The listing builds one solid part. Answer for the finished solid, in the listing's coordinates (mm). A direction names the side the tool comes from. Give positions to 0.01 mm unless a question says otherwise; leave off trailing zeros. Order: outer loops, then holes, each group sorted by start corner. A loop starts at its lowest first (then second) coordinate and runs counter-clockwise, first axis right, second up. Notation, with made-up numbers: (-28.5, -4) -> (16.5, -4) arc R22 cw to (16.5, 2) -> close; hole circle Ø8 at (69, 32.5). An arc over 180 degrees is marked (long way). Answer as a JSON object with one key per item and string values. Group by question number.
```python
from build123d import *

# Parameters (mm, degrees)
SKETCH1_W               = 203.2
SKETCH1_H               = 152.4
BOSS_EXTRUDE2_DEPTH     = 5.334
SKETCH2_R               = 17.5
CUT_EXTRUDE1_DEPTH      = 184.239656068
SKETCH3_W               = 24.13
SKETCH3_H               = 5.08
BOSS_EXTRUDE3_DEPTH     = 5.334
SKETCH4_W               = 5.842
SKETCH4_H               = 12.954
CUT_EXTRUDE2_DEPTH      = 184.239656068
MIRROR3_COPY_1_SKETCH_W = 24.13
MIRROR3_COPY_1_SKETCH_H = 5.08
MIRROR3_COPY_1_DEPTH    = 5.334


with BuildPart() as part:
    # Sketch1 → Boss-Extrude2 (new body)
    with BuildSketch(Plane(origin=(0, 0, 0), x_dir=(0, 0, -1), z_dir=(1, 0, 0))):
        with Locations((0, 76.2)):
            Rectangle(SKETCH1_W, SKETCH1_H)
    extrude(amount=BOSS_EXTRUDE2_DEPTH)

    # Sketch2 → Cut-Extrude1 (cut, through all)
    with BuildSketch(Plane.ZY):
        with Locations((0, 76.2)):
            Circle(SKETCH2_R)
    extrude(amount=-CUT_EXTRUDE1_DEPTH, mode=Mode.SUBTRACT)

    # Sketch3 → Boss-Extrude3 (add, through all)
    with BuildSketch(Plane.ZY):
        with Locations((69.85, -2.54)):
            Rectangle(SKETCH3_W, SKETCH3_H)
    boss_extrude3 = extrude(amount=-BOSS_EXTRUDE3_DEPTH)

    # Mirror1: Boss-Extrude3 across plane
    add(boss_extrude3.mirror(Plane.XY))

    # Sketch4 → Cut-Extrude2 (cut, through all)
    with BuildSketch(Plane.ZY):
        with Locations((73.025, 53.9115)):
            Rectangle(SKETCH4_W, SKETCH4_H)
        with Locations((73.025, 25.3365)):
            Rectangle(SKETCH4_W, SKETCH4_H)
    cut_extrude2 = extrude(amount=-CUT_EXTRUDE2_DEPTH, mode=Mode.SUBTRACT)

    # Mirror2: Cut-Extrude2 across plane
    add(cut_extrude2.mirror(Plane.XY), mode=Mode.SUBTRACT)

    # Mirror3: Boss-Extrude3 across plane
    add(boss_extrude3.mirror(Plane.ZX.offset(76.2)))

    # Mirror3 copy 1 sketch → Mirror3 copy 1 (add, through all)
    with BuildSketch(Plane(origin=(0, 152.4, 0), x_dir=(0, 0, -1), z_dir=(-1, 0, 0))):
        with Locations((69.85, -2.54)):
            Rectangle(MIRROR3_COPY_1_SKETCH_W, MIRROR3_COPY_1_SKETCH_H)
    extrude(amount=-MIRROR3_COPY_1_DEPTH)


solid = part.part
```
(1) A cutting plane is placed at B-B (z = 0). Determine the outline of the cut face in (x, y), and give its area (3 significant figures).
(2) For a pull along Y with two mould halves and no side action, classify faces 6 (the flat face through (3, -5.08, -70)), 7 (the flat face through (3, 152.4, -92)), 8 (the flat face through (3, 54, 70.104)) as +Y half, -Y half, draft (parallel to the pull), parting line (faces both ways), or undercut.
(3) Flat-ended cylindrical pins translate along their axes: pin 1 Ø1.6 at (x, z) = (4, 94.5) entering from +Y; pin 2 Ø1.5 at (x, y) = (3, -2) entering from -Z (3 decimals). Find the tip coordinate at first contact, or state that the pin passes through.
(4) Find the intervals of material crossed by line 1 along Z through (x, y) = (0.75, 21); line 2 along Y through (x, z) = (3.2, 0); line 3 along Y through (x, z) = (4.95, 72), in increasing order. Write a range as [from, to].
(5) Which of the six approach directions +Z, -Z, +X, -X, +Y, -Y give full straight-line access (tool end or side, diameter ignored) to faces 1 (the flat face through (3, 0, 1)), 2 (the flat face through (3, -3, -81.915)), 3 (the flat face through (3, 0, 92)), 4 (the flat face through (3, 152.4, 1)), 5 (the flat face through (3, 47.434, 73))?
(6) A cutting plane is placed at C-C (y = 76.2). Determine the outline of the cut face in (x, z), and give its area (3 significant figures).
(7) A cutting plane is placed at D-D (x = 3.85). State how many separate pieces and enclosed holes the cut face has, and give its area (3 significant figures).
(8) A cutting plane is placed at A-A (y = 53). Determine the outline of the cut face in (x, z), and give its area (3 significant figures).
Check sheet entries:
{
 "1": {"outline": "(0, 0) -> (5.33, 0) -> (5.33, 58.7) -> (0, 58.7) -> close; (0, 93.7) -> (5.33, 93.7) -> (5.33, 152.4) -> (0, 152.4) -> close", "area": "626 mm2"},
 "2": {"face 6": "-Y half", "face 7": "+Y half", "face 8": "undercut"},
 "3": {"pin 1": "stops at y = 152.4", "pin 2": "stops at z = -81.915"},
 "4": {"line 1": "z = [-101.6, -75.95], [-70.1, 70.1], [75.95, 101.6]", "line 2": "y = [0, 58.7], [93.7, 152.4]", "line 3": "y = [-5.08, 18.86], [31.81, 47.43], [60.39, 157.48]"},
 "5": {"face 1": "+X, -X, -Y", "face 2": "-Z, +X, -X, -Y", "face 3": "+Z, +X, -X, -Y", "face 4": "+X, -X, +Y", "face 5": "+X, -X"},
 "6": {"outline": "(0, -101.6) -> (5.33, -101.6) -> (5.33, -17.5) -> (0, -17.5) -> close; (0, 17.5) -> (5.33, 17.5) -> (5.33, 101.6) -> (0, 101.6) -> close", "area": "897 mm2"},
 "7": {"separate pieces": "1", "enclosed holes": "5", "area": "30,200 mm2"},
 "8": {"outline": "(0, -101.6) -> (5.33, -101.6) -> (5.33, -75.95) -> (0, -75.95) -> close; (0, -70.1) -> (5.33, -70.1) -> (5.33, 70.1) -> (0, 70.1) -> close; (0, 75.95) -> (5.33, 75.95) -> (5.33, 101.6) -> (0, 101.6) -> close", "area": "1,020 mm2"}
}
